Design review of the part built by this model. Coordinates are the model's own, in mm. Give positions to 0.01 mm unless a question says otherwise; leave off trailing zeros. Loops run counter-clockwise (first coordinate to the right, second up) from the corner with the lowest first, then second, coordinate; pieces in that order, holes last.
from build123d import *

# Parameters (mm, degrees)
SKETCH1_R           = 428.5
SKETCH1_R_2         = 90
BOSS_EXTRUDE1_DEPTH = 6
SKETCH2_R           = 3
CUT_EXTRUDE1_DEPTH  = 6
SKETCH5_R           = 5
BOSS_EXTRUDE2_DEPTH = 35
CIRPATTERN1_COUNT   = 6
CIRPATTERN2_COUNT   = 4


with BuildPart() as part:
    # Sketch1 → Boss-Extrude1 (new body)
    with BuildSketch(Plane(origin=(0, 0, 0), x_dir=(1, 0, 0), z_dir=(0, 1, 0))):
        with Locations(Location((0, 0, 0), (0, 0, 270))):
            Circle(SKETCH1_R)
        with Locations(Location((0, 0, 0), (0, 0, 270))):
            Circle(SKETCH1_R_2, mode=Mode.SUBTRACT)
    extrude(amount=BOSS_EXTRUDE1_DEPTH)

    # Sketch2 → Cut-Extrude1 (cut)
    with BuildSketch(Plane(origin=(0, 6, 0), x_dir=(1, 0, 0), z_dir=(0, 1, 0))):
        with Locations(Location((0, 157.5, 0), (0, 0, 270))):
            Circle(SKETCH2_R)
    cut_extrude1 = extrude(amount=-CUT_EXTRUDE1_DEPTH, mode=Mode.SUBTRACT)

    # Sketch5 → Boss-Extrude2 (add)
    with BuildSketch(Plane(origin=(0, 6, 0), x_dir=(1, 0, 0), z_dir=(0, 1, 0))):
        with Locations(Location((93.691648507, 93.691648507, 0), (0, 0, 270))):
            Circle(SKETCH5_R)
    boss_extrude2 = extrude(amount=BOSS_EXTRUDE2_DEPTH)

    # CirPattern1: Cut-Extrude1 ×6 about axis
    cirpattern1_axis = Axis((0, 0, 0), (0, 1, 0))
    for i in range(1, CIRPATTERN1_COUNT):
        add(cut_extrude1.rotate(cirpattern1_axis, i * 360 / CIRPATTERN1_COUNT), mode=Mode.SUBTRACT)

    # CirPattern2: Boss-Extrude2 ×4 about axis
    cirpattern2_axis = Axis((0, 0, 0), (0, 1, 0))
    for i in range(1, CIRPATTERN2_COUNT):
        add(boss_extrude2.rotate(cirpattern2_axis, i * 360 / CIRPATTERN2_COUNT))


solid = part.part
Q1. Wall thickness on line 1 (X direction, y = 3.55, z = 78.75); line 2 (Y direction, x = -208.5, z = 320.5); line 3 (X direction, y = 3, z = 78): over which ranges is each line inside the solid? List them lowest first.
Results:
line 1: x = -421.2 to -139.4, -133.4 to -43.57, 43.57 to 133.4, 139.4 to 421.2
line 2: y = 0 to 6
line 3: x = -421.34 to -139.3, -133.49 to -44.9, 44.9 to 133.49, 139.3 to 421.34
Q2. Take a section at B-B (y = 19.5). Give the boundary of the cut face in (x, z), plus the area to 3 significant figures.
Results:
outline: circle Ø10 at (-93.69, -93.69); circle Ø10 at (-93.69, 93.69); circle Ø10 at (93.69, -93.69); circle Ø10 at (93.69, 93.69)
area: 314 mm2
Q3. Draft analysis for pull direction X (two halves, no side actions). For faces 1 (the face through (6, 0, -101)), 2 (the face through (-260.74, 2.96, -340.04)), 3 (the face through (-34.471, 2.958, 83.137)), state which applies: pulls with the +X half, pulls with the -X half, needs draft (parallel to the pull), parting line crosses it, or undercut.
Results:
face 1: needs draft
face 2: parting line crosses it
face 3: undercut
Q4. Insertion check: pin 1 (9.5 mm diameter, centred on x = 0, z = 157.5, fed in from +Y); pin 2 (10 mm diameter, centred on y = 6.5, z = 336.5, fed in from -X). Each pin has a flat end and moves straight along its axis. Give the tip position at first contact, or say it passes through.
Results:
pin 1: stops at y = 6
pin 2: stops at x = -271.48
Q5. Take a section at D-D (x = 351.5). Give the boundary of the cut face in (y, z), plus the area to 3 significant figures.
Results:
outline: (0, -245.07) - (6, -245.07) - (6, 245.07) - (0, 245.07) - close
area: 2,940 mm2
Q6. Take a section at C-C (z = 360). Give the boundary of the cut face in (x, y).
Results:
outline: (-232.41, 0) - (232.41, 0) - (232.41, 6) - (-232.41, 6) - close
Q7. Take a section at A-A (x = 24). Give the boundary of the cut face in (y, z), plus the area to 3 significant figures.
Results:
outline: (0, -427.83) - (6, -427.83) - (6, -86.74) - (0, -86.74) - close; (0, 86.74) - (6, 86.74) - (6, 427.83) - (0, 427.83) - close
area: 4,090 mm2
